CAD build for the part. Positions are in the model's coordinates, mm. A direction names the side the tool comes from. Coordinates: 2 decimals unless noted, no trailing zeros. Write each loop counter-clockwise with the first axis right and the second up, starting at its lowest first coordinate (ties: lowest second). Pieces come first, ordered by that corner, then holes. Notation, with made-up numbers: (79, -18) - (100, -18) arc R17 ccw to (100, 5) - close; hole circle Ø3 at (43.25, 76.5). An arc over 180 degrees is marked (long way). Answer in a Markdown table with one row per item. Add a question column.
Q1. Band-saw the part on B-B (x = 2.5). List the corners of the cut face in (y, z), and give its area (3 significant figures).
Q2. Drill centre lines: line 1 along Z through (x, y) = (27, 9.5); line 2 along Z through (x, y) = (44, 5.3); line 3 along Z through (x, y) = (-17.5, 4). Where is each one in solid material? Low to high. Write a range as from..to.
Q3. Two-plate mould, pull along X, no slides. Class faces 1 (the cylindrical face through (26, 9.4, 7)), 2 (the flat face through (34, 4.3, -11)), 3 (the flat face through (13, 5, -7.5)): +X half, -X half, draft (parallel to the pull), parting line (faces both ways), or undercut.
Q4. 3-axis set-ups, long thin cutter, end or side, ignore diameter. For faces 4 (the flat face through (-48, 4, 6)), 5 (the flat face through (-32.1, 5, -10)), 6 (the flat face through (-37, 3.7, 14)): which of +Z, -Z, +X, -X, +Y, -Y reach the whole face in a straight line?
Q5. Pin check, flat tips, straight feed: pin 1 (1.2 mm diameter, centred on x = 34, z = 0, fed in from -Y); pin 2 (9.5 mm diameter, centred on x = -7, z = 3.5, fed in from -Y); pin 3 (3 mm diameter, centred on x = -42.5, z = -9, fed in from -Y); pin 4 (0.6 mm diameter, centred on x = -48, z = -2, fed in from -Y). Stop position of each tip, or through.
Q6. Band-saw the part on A-A (x = -11.5). List the corners of the cut face in (y, z), and give its area (3 significant figures).
```python
from build123d import *

# Parameters (mm, degrees)
SKETCH_1_W           = 96
SKETCH_1_H           = 30.2
EXTRUDE_1_DEPTH      = 9.8
SKETCH_1_8_W         = 0.1
SKETCH_1_8_H         = 26.2
SKETCH_1_8_W_2       = 94
CUT_EXTRUDE_2_DEPTH  = 4.3
SKETCH_2_R           = 12.7
CUT_EXTRUDE_3_DEPTH  = 4.8
SKETCH_3_W           = 32.4
SKETCH_3_H           = 19.2
CUT_EXTRUDE_4_DEPTH  = 4.8
SKETCH_4_R           = 0.6
CUT_EXTRUDE_5_DEPTH  = 2
SKETCH_5_W           = 7.8
SKETCH_5_H           = 2
SKETCH_5_W_2         = 15.6
CUT_EXTRUDE_6_DEPTH  = 3.7
SKETCH_6_R           = 0.4
CUT_EXTRUDE_7_DEPTH  = 2
SKETCH_7_W           = 12
SKETCH_7_H           = 6.9
SKETCH_7_W_2         = 20
SKETCH_7_H_2         = 2
CUT_EXTRUDE_9_DEPTH  = 1.9
SKETCH_8_W           = 4.8
SKETCH_8_H           = 9.7
CUT_EXTRUDE_10_DEPTH = 2
OTHER_START          = 9.1
OTHER_1_OUTLINE_R    = 1
OTHER_1_DEPTH        = 0.7


# Read off the part's stored shape, not the designer's step: 填充阵列1
with BuildPart() as part:
    # 草图1 → 凸台-拉伸1 (new body)
    with BuildSketch(Plane(origin=(0, 0, 0), x_dir=(1, 0, 0), z_dir=(0, 1, 0))):
        with Locations((-1, 0)):
            Rectangle(SKETCH_1_W, SKETCH_1_H)
    extrude(amount=EXTRUDE_1_DEPTH)

    # 草图1<8> → 切除-拉伸2 (cut)
    with BuildSketch(Plane(origin=(0, 0, 0), x_dir=(1, 0, 0), z_dir=(0, 1, 0))):
        with Locations((-47.05, 0)):
            Rectangle(SKETCH_1_8_W, SKETCH_1_8_H)
        Rectangle(SKETCH_1_8_W_2, SKETCH_1_8_H)
    extrude(amount=CUT_EXTRUDE_2_DEPTH, mode=Mode.SUBTRACT)

    # 草图2 → 切除-拉伸3 (cut)
    with BuildSketch(Plane(origin=(0, 4.3, 0), x_dir=(-1, 0, 0), z_dir=(0, -1, 0))):
        with Locations(Location((-27, 0, 0), (0, 0, 90))):
            Circle(SKETCH_2_R)
    extrude(amount=-CUT_EXTRUDE_3_DEPTH, mode=Mode.SUBTRACT)

    # 草图3 → 切除-拉伸4 (cut)
    with BuildSketch(Plane.XZ.offset(-4.3)):
        with Locations((-6.9, 0)):
            Rectangle(SKETCH_3_W, SKETCH_3_H)
    extrude(amount=-CUT_EXTRUDE_4_DEPTH, mode=Mode.SUBTRACT)

    # 草图4 → 切除-拉伸5 (cut)
    with BuildSketch(Plane.XZ.offset(-4.3)):
        Polygon((-23.1, 7.5), (-47.1, 7.5), (-47.1, -7.5), (-32.1, -7.5), (-32.1, -13.1), (-7.1, -13.1), (-7.1, -9.6), (-23.1, -9.6), align=None)
        with BuildLine():
            Line((37, 13.1), (14, 13.1))
            Line((14, 13.1), (14, 10.1))
            Line((14, 10.1), (19.300649378, 10.1))
            ThreePointArc((19.300649378, 10.1), (27, 12.7), (34.699350622, 10.1))
            Line((34.699350622, 10.1), (37, 10.1))
            Line((37, 10.1), (37, 13.1))
        make_face()
        with BuildLine():
            Line((16.75109762, 7.5), (9.3, 7.5))
            Line((9.3, 7.5), (9.3, -7.5))
            Line((9.3, -7.5), (16.75109762, -7.5))
            ThreePointArc((16.75109762, -7.5), (14.3, 0), (16.75109762, 7.5))
        make_face()
        with Locations(Location((-44, 10, 0), (0, 0, 270))):
            Circle(SKETCH_4_R)
        with Locations(Location((-44, -10, 0), (0, 0, 270))):
            Circle(SKETCH_4_R)
        with Locations(Location((44, 10, 0), (0, 0, 270))):
            Circle(SKETCH_4_R)
        with Locations(Location((44, -10, 0), (0, 0, 270))):
            Circle(SKETCH_4_R)
    extrude(amount=-CUT_EXTRUDE_5_DEPTH, mode=Mode.SUBTRACT)

    # 草图5 → 切除-拉伸6 (cut)
    with BuildSketch(Plane.XZ):
        with Locations((-37.2, 14.1)):
            Rectangle(SKETCH_5_W, SKETCH_5_H)
        with Locations((32.9, 14.1)):
            Rectangle(SKETCH_5_W_2, SKETCH_5_H)
    extrude(amount=-CUT_EXTRUDE_6_DEPTH, mode=Mode.SUBTRACT)

    # 草图6 → 切除-拉伸7 (cut)
    with BuildSketch(Plane.ZY.offset(49)):
        with Locations((-8.05, 4.9)):
            Circle(SKETCH_6_R)
        with Locations((8.05, 4.9)):
            Circle(SKETCH_6_R)
    extrude(amount=-CUT_EXTRUDE_7_DEPTH, mode=Mode.SUBTRACT)

    # 草图7 → 切除-拉伸9 (cut)
    with BuildSketch(Plane.ZY.offset(49)):
        with Locations((0, 3.45)):
            Rectangle(SKETCH_7_W, SKETCH_7_H)
        with Locations((0, 1)):
            Rectangle(SKETCH_7_W_2, SKETCH_7_H_2)
    extrude(amount=-CUT_EXTRUDE_9_DEPTH, mode=Mode.SUBTRACT)

    # 草图8 → 切除-拉伸10 (cut)
    with BuildSketch(Plane.XZ.offset(-6.3)):
        with Locations((-44.7, 2.65)):
            Rectangle(SKETCH_8_W, SKETCH_8_H)
    extrude(amount=-CUT_EXTRUDE_10_DEPTH, mode=Mode.SUBTRACT)

    # 填充阵列1 outline → 填充阵列1 (cut)
    with BuildSketch(Plane(origin=(0, 0, 0), x_dir=(1, 0, 0), z_dir=(0, 1, 0)).offset(OTHER_START)):
        with Locations((27, -3.369e-06)):
            Circle(OTHER_1_OUTLINE_R)
        with Locations((22.050252532, 4.949744099)):
            Circle(OTHER_1_OUTLINE_R)
        with Locations((33.876037706, 7.935367161)):
            Circle(OTHER_1_OUTLINE_R)
        with Locations((20.532843272, 2.678780657)):
            Circle(OTHER_1_OUTLINE_R)
        with Locations((31.361857637, 9.551132582)):
            Circle(OTHER_1_OUTLINE_R)
        with Locations((27, 6.999996631)):
            Circle(OTHER_1_OUTLINE_R)
        with Locations((37.074676223, 2.958188477)):
            Circle(OTHER_1_OUTLINE_R)
        with Locations((24.321215973, 6.467153358)):
            Circle(OTHER_1_OUTLINE_R)
        with Locations((35.833162095, 5.676725214)):
            Circle(OTHER_1_OUTLINE_R)
        with Locations((28.494305802, 10.39312177)):
            Circle(OTHER_1_OUTLINE_R)
        with Locations((25.505694198, 10.39312177)):
            Circle(OTHER_1_OUTLINE_R)
        with Locations((22.638142363, 9.551132582)):
            Circle(OTHER_1_OUTLINE_R)
        with Locations((20.123962294, 7.935367161)):
            Circle(OTHER_1_OUTLINE_R)
        with Locations((18.166837905, 5.676725214)):
            Circle(OTHER_1_OUTLINE_R)
        with Locations((16.925323777, 2.958188477)):
            Circle(OTHER_1_OUTLINE_R)
        with Locations((20.123962294, -7.9353739)):
            Circle(OTHER_1_OUTLINE_R)
        with Locations((24.321215973, -6.467160097)):
            Circle(OTHER_1_OUTLINE_R)
        with Locations((29.474873734, -2.474877104)):
            Circle(OTHER_1_OUTLINE_R)
        with Locations((18.166837905, -5.676731953)):
            Circle(OTHER_1_OUTLINE_R)
        with Locations((29.474873734, 2.474870365)):
            Circle(OTHER_1_OUTLINE_R)
        with Locations((22.638142363, -9.551139321)):
            Circle(OTHER_1_OUTLINE_R)
        with Locations((27, -7.000003369)):
            Circle(OTHER_1_OUTLINE_R)
        with Locations((30.5, -3.369e-06)):
            Circle(OTHER_1_OUTLINE_R)
        with Locations((24.525126266, -2.474877104)):
            Circle(OTHER_1_OUTLINE_R)
        with Locations((16.5, -3.369e-06)):
            Circle(OTHER_1_OUTLINE_R)
        with Locations((20, -3.369e-06)):
            Circle(OTHER_1_OUTLINE_R)
        with Locations((23.5, -3.369e-06)):
            Circle(OTHER_1_OUTLINE_R)
        with Locations((22.050252532, -4.949750838)):
            Circle(OTHER_1_OUTLINE_R)
        with Locations((27, -3.500003369)):
            Circle(OTHER_1_OUTLINE_R)
        with Locations((16.925323777, -2.958195216)):
            Circle(OTHER_1_OUTLINE_R)
        with Locations((20.532843272, -2.678787396)):
            Circle(OTHER_1_OUTLINE_R)
        with Locations((35.833162095, -5.676731953)):
            Circle(OTHER_1_OUTLINE_R)
        with Locations((33.467156728, 2.678780657)):
            Circle(OTHER_1_OUTLINE_R)
        with Locations((33.876037706, -7.9353739)):
            Circle(OTHER_1_OUTLINE_R)
        with Locations((34, -3.369e-06)):
            Circle(OTHER_1_OUTLINE_R)
        with Locations((37.5, -3.369e-06)):
            Circle(OTHER_1_OUTLINE_R)
        with Locations((29.678784027, 6.467153358)):
            Circle(OTHER_1_OUTLINE_R)
        with Locations((37.074676223, -2.958195216)):
            Circle(OTHER_1_OUTLINE_R)
        with Locations((31.949747468, 4.949744099)):
            Circle(OTHER_1_OUTLINE_R)
        with Locations((31.949747468, -4.949750838)):
            Circle(OTHER_1_OUTLINE_R)
        with Locations((27, 3.499996631)):
            Circle(OTHER_1_OUTLINE_R)
        with Locations((25.505694198, -10.393128509)):
            Circle(OTHER_1_OUTLINE_R)
        with Locations((29.678784027, -6.467160097)):
            Circle(OTHER_1_OUTLINE_R)
        with Locations((28.494305802, -10.393128509)):
            Circle(OTHER_1_OUTLINE_R)
        with Locations((24.525126266, 2.474870365)):
            Circle(OTHER_1_OUTLINE_R)
        with Locations((33.467156728, -2.678787396)):
            Circle(OTHER_1_OUTLINE_R)
        with Locations((31.361857637, -9.551139321)):
            Circle(OTHER_1_OUTLINE_R)
    extrude(amount=OTHER_1_DEPTH, mode=Mode.SUBTRACT)


solid = part.part
```
Checked values:
| question | item | result |
|---|---|---|
| 1 | outline | (0, -15.1) - (9.8, -15.1) - (9.8, 15.1) - (0, 15.1) - (0, 13.1) - (4.3, 13.1) - (4.3, 9.6) - (9.1, 9.6) - (9.1, -9.6) - (4.3, -9.6) - (4.3, -13.1) - (0, -13.1) - close |
| 1 | area | 91.1 mm² |
| 2 | line 1 | z = -15.1..-8, -6..-4.5, -2.5..-1, 1..2.5, 4.5..6, 8..15.1 |
| 2 | line 2 | z = -15.1..-10.6, -9.4..9.4, 10.6..15.1 |
| 2 | line 3 | z = -15.1..-13.1, 13.1..15.1 |
| 3 | face 1 | undercut |
| 3 | face 2 | draft |
| 3 | face 3 | undercut |
| 4 | face 4 | -X, -Y |
| 4 | face 5 | -Y |
| 4 | face 6 | +Z, -Y |
| 5 | pin 1 | passes through |
| 5 | pin 2 | stops at y = 9.1 |
| 5 | pin 3 | stops at y = 4.3 |
| 5 | pin 4 | stops at y = 6.9 |
| 6 | outline | (0, -15.1) - (9.8, -15.1) - (9.8, 15.1) - (0, 15.1) - (0, 13.1) - (4.3, 13.1) - (4.3, 9.6) - (9.1, 9.6) - (9.1, -9.6) - (6.3, -9.6) - (6.3, -13.1) - (0, -13.1) - close |
| 6 | area | 84.1 mm² |
